Input: dimensioned drawing with shaded views. Units: mm. Origin: part minimum x, y, z. Coordinates: 2 decimals unless noted, no trailing zeros. Loops run counter-clockwise (first coordinate to the right, second up) from the corner with the lowest first, then second, coordinate; pieces in that order, holes last.
(1) Section A-A, the plane x = 19.5. Return loops of the section in (y, z) (1 decimal), then the cut area to 3 significant figures.
(2) Line query: L1, parallel to Z at x = 111.5, y = 2.7; L2, parallel to Z at x = 74, y = 2.55; L3, parallel to Z at x = 29, y = 2.85. Output: solid intervals per line, ascending.
(3) Section C-C, the plane z = 22. Return loops of the section in (x, y) (1 decimal), then the cut area to 3 significant figures.
(4) Contact query for flat-ended pins moving along their axis: P1, Ø1.5, axis at y = 1.5, z = 10, coming from the +X side; P2, Ø1, axis at x = 99, y = 1, coming from the -Z side. Output: stop coordinate, or through.
(5) Section B-B, the plane y = 1.2. Give the number of separate pieces and of enclosed holes in the cut face, then the cut area to 3 significant figures.
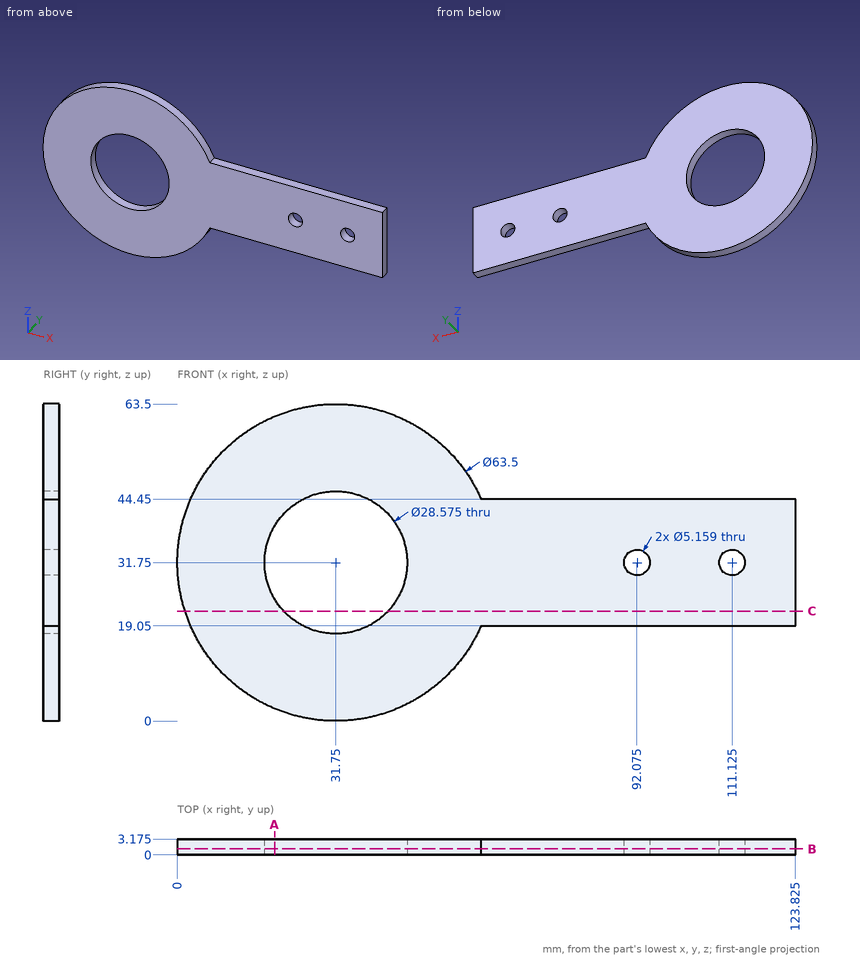
Report:
1. outline: (0, 2.5) - (3.2, 2.5) - (3.2, 24.4) - (0, 24.4) - close; (0, 39.1) - (3.2, 39.1) - (3.2, 61) - (0, 61) - close
1. area: 139 mm2
2. L1: z = 19.05 to 29.2, 34.3 to 44.45
2. L2: z = 19.05 to 44.45
2. L3: z = 0.12 to 17.73, 45.77 to 63.38
3. outline: (1.5, 0) - (21.3, 0) - (21.3, 3.2) - (1.5, 3.2) - close; (42.2, 0) - (123.8, 0) - (123.8, 3.2) - (42.2, 3.2) - close
3. area: 322 mm2
4. P1: stops at x = 55.56
4. P2: stops at z = 19.05
5. separate pieces: 1
5. enclosed holes: 3
5. area: 4,040 mm2
